```python
from build123d import *

# Parameters (mm, degrees)
SKETCH1_W           = 50.8
SKETCH1_H           = 203.2
BOSS_EXTRUDE2_DEPTH = 38.1
SKETCH2_R           = 9.525
CUT_EXTRUDE1_DEPTH  = 38.1
SKETCH3_R           = 9.525
CUT_EXTRUDE2_DEPTH  = 38.1
SKETCH4_W           = 253.975113334
SKETCH4_H           = 254.028971003
CUT_EXTRUDE3_DEPTH  = 7.62
SKETCH5_W           = 254
SKETCH5_H           = 254.028971003
CUT_EXTRUDE4_DEPTH  = 60.96
SKETCH6_W           = 50.8
SKETCH6_H           = 50.828971003
BOSS_EXTRUDE3_DEPTH = 7.62
CHAMFER1_SIZE       = 7.62


with BuildPart() as part:
    # Sketch1 → Boss-Extrude2 (new body)
    with BuildSketch(Plane(origin=(0, 0, 0), x_dir=(1, 0, 0), z_dir=(0, 1, 0))):
        Polygon((0, 0), (0, 25.4), (-50.8, 25.4), (-101.6, 25.4), (-152.4, 25.4), (-203.2, 25.4), (-203.2, 228.6), (-228.6, 228.6), (-228.6, 0), align=None)
        with Locations((-127, 127)):
            Rectangle(SKETCH1_W, SKETCH1_H)
        with Locations((-25.4, 127)):
            Rectangle(SKETCH1_W, SKETCH1_H)
    extrude(amount=BOSS_EXTRUDE2_DEPTH)

    # Sketch2 → Cut-Extrude1 (cut)
    with BuildSketch(Plane(origin=(0, 0, -228.6), x_dir=(-1, 0, 0), z_dir=(0, 0, -1))):
        with Locations((215.9, 19.05)):
            Circle(SKETCH2_R)
    extrude(amount=-CUT_EXTRUDE1_DEPTH, mode=Mode.SUBTRACT)

    # Sketch3 → Cut-Extrude2 (cut)
    with BuildSketch(Plane(origin=(0, 0, 0), x_dir=(0, 0, -1), z_dir=(1, 0, 0))):
        with Locations((12.728971003, 19.05)):
            Circle(SKETCH3_R)
    extrude(amount=-CUT_EXTRUDE2_DEPTH, mode=Mode.SUBTRACT)

    # Sketch4 → Cut-Extrude3 (cut)
    with BuildSketch(Plane(origin=(0, 7.62, 0), x_dir=(-1, 0, 0), z_dir=(0, -1, 0))):
        with Locations((-50.812443333, 304.785514498)):
            Rectangle(SKETCH4_W, SKETCH4_H)
    extrude(amount=-CUT_EXTRUDE3_DEPTH, mode=Mode.SUBTRACT)

    # Sketch5 → Cut-Extrude4 (cut)
    with BuildSketch(Plane.XZ.offset(-7.62)):
        with Locations((50.8, -304.785514498)):
            Rectangle(SKETCH5_W, SKETCH5_H)
    extrude(amount=CUT_EXTRUDE4_DEPTH, mode=Mode.SUBTRACT)

    # Sketch6 → Boss-Extrude3 (add)
    with BuildSketch(Plane(origin=(0, 15.24, 0), x_dir=(-1, 0, 0), z_dir=(0, -1, 0))):
        with Locations((25.4, 203.185514499)):
            Rectangle(SKETCH6_W, SKETCH6_H)
    extrude(amount=BOSS_EXTRUDE3_DEPTH)

    # Chamfer1
    chamfer1_edges = [part.edges().sort_by_distance(p)[0] for p in [
        (-114.3, 0, 0),
        (-228.6, 0, -114.3),
        (-228.6, 38.1, -114.3),
        (-114.3, 38.1, 0),
    ]]
    chamfer(chamfer1_edges, length=CHAMFER1_SIZE)


solid = part.part
```
Check sheet for the modelled part. Datum: model origin and axes. Units: mm. A direction names the side the tool comes from. Give positions to 0.01 mm unless a question says otherwise; leave off trailing zeros. Order: outer loops, then holes, each group sorted by start corner. A loop starts at its lowest first (then second) coordinate and runs counter-clockwise, first axis right, second up. Notation, with made-up numbers: M -34.5,-21 L 7.5,-21 A13 ccw 7.5,-8 Z; hole C -25,38.5 d5. An arc over 180 degrees is marked long. Answer in a Markdown table with one row per item.
1) Release check for a two-part mould opening along Z. For faces 1 (the flat face through (-115.9, 3.86, -3.76)), 2 (the flat face through (-50.8, 19, -126)), 3 (the flat face through (-38.1, 19, -13)), 4 (the flat face through (-26, 4, -177.771)) record: +Z half, -Z half, draft (parallel to the pull), parting line (faces both ways), or undercut.
Filled sheet:
| item | result |
|---|---|
| face 1 | +Z half |
| face 2 | draft |
| face 3 | undercut |
| face 4 | -Z half |
2) Cross-section at A-A, the plane z = -155.5. Enter the section's corners in (x, y), plus the area to 3 significant figures.
Filled sheet:
| item | result |
|---|---|
| outline | M -228.6,7.62 L -220.98,0 L -203.2,0 L -203.2,38.1 L -220.98,38.1 L -228.6,30.48 Z; M -152.4,0 L -101.6,0 L -101.6,38.1 L -152.4,38.1 Z; M -50.8,0 L 0,0 L 0,38.1 L -50.8,38.1 Z |
| area | 4,780 mm2 |
3) Thickness scan on L1, parallel to X at y = 19, z = -217; L2, parallel to X at y = 14, z = -189; L3, parallel to Z at x = -20, y = 19. Record the ranges inside material, lowest first. Write a range as [from, to].
Filled sheet:
| item | result |
|---|---|
| L1 | x = [-228.6, -225.42], [-206.38, -203.2], [-152.4, -101.6], [-50.8, 0] |
| L2 | x = [-228.6, -203.2], [-152.4, -101.6], [-50.8, 0] |
| L3 | z = [-228.6, -22.25], [-3.2, 0] |
4) Cross-section at C-C, the plane x = -76. Enter the section's corners in (y, z).
Filled sheet:
| item | result |
|---|---|
| outline | M 0,-25.4 L 38.1,-25.4 L 38.1,-7.62 L 30.48,0 L 7.62,0 L 0,-7.62 Z |
5) Gauge pin test, flat ends, axial feed: P1, Ø8.5, axis at x = -14.5, y = 3.5, coming from the -Z side; P2, Ø2, axis at y = 33, z = -141, coming from the -X side; P3, Ø19, axis at x = -68.5, y = 16, coming from the -Z side; P4, Ø15, axis at x = -215.9, y = 19.05, coming from the -Z side. Record the tip position at first contact, or that the pin passes through.
Filled sheet:
| item | result |
|---|---|
| P1 | stops at z = -228.6 |
| P2 | stops at x = -227.08 |
| P3 | stops at z = -25.4 |
| P4 | stops at z = -190.5 |
6) Cross-section at D-D, the plane x = -215.9. Enter the section's corners in (y, z) (3 decimals), plus the area to 3 significant figures.
Filled sheet:
| item | result |
|---|---|
| outline | M 0,-228.6 L 9.525,-228.6 L 9.525,-190.5 L 28.575,-190.5 L 28.575,-228.6 L 38.1,-228.6 L 38.1,-7.62 L 30.48,0 L 7.62,0 L 0,-7.62 Z |
| area | 7,930 mm2 |
7) Cross-section at B-B, the plane y = 19.05. Enter the section's corners in (x, z) (3 decimals), plus the area to 3 significant figures.
Filled sheet:
| item | result |
|---|---|
| outline | M -228.6,-228.6 L -225.425,-228.6 L -225.425,-190.5 L -206.375,-190.5 L -206.375,-228.6 L -203.2,-228.6 L -203.2,-25.4 L -152.4,-25.4 L -152.4,-228.6 L -101.6,-228.6 L -101.6,-25.4 L -50.8,-25.4 L -50.8,-228.6 L 0,-228.6 L 0,-22.254 L -38.1,-22.254 L -38.1,-3.204 L 0,-3.204 L 0,0 L -228.6,0 Z |
| area | 30,200 mm2 |
8) Access from +Z, -Z, +X, -X, +Y, -Y to the whole of each face (thin tool, end or side, straight path). Record for faces 5 (the flat face through (-25, 23, -228.6)), 6 (the cylindrical face through (-224.7, 15.4, -209.8)), 7 (the flat face through (-76, 19, -25.4)), 8 (the flat face through (0, 19, -113)), 9 (the flat face through (-25, 7.62, -204)).
Filled sheet:
| item | result |
|---|---|
| face 5 | -Z, +X, -X, +Y, -Y |
| face 6 | -Z |
| face 7 | -Z, +Y, -Y |
| face 8 | +Z, -Z, +X, +Y, -Y |
| face 9 | -Z, +X, -Y |
